The model under review builds one solid part; all positions refer to its coordinate system, in mm. Coordinates: 2 decimals unless noted, no trailing zeros. Order: outer loops, then holes, each group sorted by start corner. A loop starts at its lowest first (then second) coordinate and runs counter-clockwise, first axis right, second up. Notation, with made-up numbers: M -14.75,40 L 12.25,40 A20 ccw 12.25,51 Z; hole C 20.5,52.25 d2. An arc over 180 degrees is marked long. One line per item, written item: value.
```python
from build123d import *

# Parameters (mm, degrees)
SKETCH1_R           = 117.5
SKETCH1_R_2         = 10.25
SKETCH1_R_3         = 12.5
SKETCH1_R_4         = 1.75
BOSS_EXTRUDE1_DEPTH = 1.5


with BuildPart() as part:
    # Sketch1 → Boss-Extrude1 (new, symmetric)
    with BuildSketch(Plane(origin=(0, 0, 0), x_dir=(1, 0, 0), z_dir=(0, 1, 0))):
        with Locations(Location((0, 0, 0), (0, 0, 270))):
            Circle(SKETCH1_R)
        with Locations(Location((0, 0, 0), (0, 0, 270))):
            Circle(SKETCH1_R_2, mode=Mode.SUBTRACT)
        with Locations(Location((0, 70, 0), (0, 0, 270))):
            Circle(SKETCH1_R_3, mode=Mode.SUBTRACT)
        with Locations(Location((70, 0, 0), (0, 0, 270))):
            Circle(SKETCH1_R_3, mode=Mode.SUBTRACT)
        with Locations(Location((0, -70, 0), (0, 0, 270))):
            Circle(SKETCH1_R_3, mode=Mode.SUBTRACT)
        with Locations(Location((-70, 0, 0), (0, 0, 270))):
            Circle(SKETCH1_R_3, mode=Mode.SUBTRACT)
        with Locations(Location((0, 110, 0), (0, 0, 270))):
            Circle(SKETCH1_R_4, mode=Mode.SUBTRACT)
        with Locations(Location((77.781745931, 77.781745931, 0), (0, 0, 270))):
            Circle(SKETCH1_R_4, mode=Mode.SUBTRACT)
        with Locations(Location((110, 0, 0), (0, 0, 270))):
            Circle(SKETCH1_R_4, mode=Mode.SUBTRACT)
        with Locations(Location((77.781745931, -77.781745931, 0), (0, 0, 270))):
            Circle(SKETCH1_R_4, mode=Mode.SUBTRACT)
        with Locations(Location((0, -110, 0), (0, 0, 270))):
            Circle(SKETCH1_R_4, mode=Mode.SUBTRACT)
        with Locations(Location((-77.781745931, -77.781745931, 0), (0, 0, 270))):
            Circle(SKETCH1_R_4, mode=Mode.SUBTRACT)
        with Locations(Location((-110, 0, 0), (0, 0, 270))):
            Circle(SKETCH1_R_4, mode=Mode.SUBTRACT)
        with Locations(Location((-77.781745931, 77.781745931, 0), (0, 0, 270))):
            Circle(SKETCH1_R_4, mode=Mode.SUBTRACT)
        with Locations(Location((0, 37.5, 0), (0, 0, 270))):
            Circle(SKETCH1_R_4, mode=Mode.SUBTRACT)
        with Locations(Location((26.516504294, 26.516504294, 0), (0, 0, 270))):
            Circle(SKETCH1_R_4, mode=Mode.SUBTRACT)
        with Locations(Location((37.5, 0, 0), (0, 0, 270))):
            Circle(SKETCH1_R_4, mode=Mode.SUBTRACT)
        with Locations(Location((26.516504294, -26.516504294, 0), (0, 0, 270))):
            Circle(SKETCH1_R_4, mode=Mode.SUBTRACT)
        with Locations(Location((0, -37.5, 0), (0, 0, 270))):
            Circle(SKETCH1_R_4, mode=Mode.SUBTRACT)
        with Locations(Location((-26.516504294, -26.516504294, 0), (0, 0, 270))):
            Circle(SKETCH1_R_4, mode=Mode.SUBTRACT)
        with Locations(Location((-37.5, 0, 0), (0, 0, 270))):
            Circle(SKETCH1_R_4, mode=Mode.SUBTRACT)
        with Locations(Location((-26.516504294, 26.516504294, 0), (0, 0, 270))):
            Circle(SKETCH1_R_4, mode=Mode.SUBTRACT)
    extrude(amount=BOSS_EXTRUDE1_DEPTH, both=True)


solid = part.part
```
(1) Insertion check: pin 1 Ø5 at (x, z) = (81, -3) entering from -Y. The pin has a flat end and moves straight along its axis. Give the tip position at first contact, or say it passes through.
Geometry results:
pin 1: stops at y = -1.5
(2) We need section B-B, the plane z = -64.5. State the section outline as (x, y) points.
Geometry results:
outline: M -98.21,-1.5 L -11.22,-1.5 L -11.22,1.5 L -98.21,1.5 Z; M 11.22,-1.5 L 98.21,-1.5 L 98.21,1.5 L 11.22,1.5 Z
(3) For L1, parallel to X at y = 0.3, z = 7.5; L2, parallel to Z at x = 5, y = 0.15; L3, parallel to Z at x = 2, y = -0.5, list the stretches that pass through material, from the lowest coordinate up.
Geometry results:
L1: x = -117.26 to -80, -60 to -6.99, 6.99 to 60, 80 to 117.26
L2: z = -117.39 to -81.46, -58.54 to -8.95, 8.95 to 58.54, 81.46 to 117.39
L3: z = -117.48 to -82.34, -57.66 to -10.05, 10.05 to 57.66, 82.34 to 117.48
(4) We need section A-A, the plane x = 62.5. State the section outline as (y, z) points.
Geometry results:
outline: M -1.5,-99.5 L 1.5,-99.5 L 1.5,-10 L -1.5,-10 Z; M -1.5,10 L 1.5,10 L 1.5,99.5 L -1.5,99.5 Z
(5) Mouldability with a two-part tool opening along Z and no side actions: class faces 1 (the flat face through (-24, 1.5, -2)), 2 (the cylindrical face through (0.55, -0.021, -82.488)), 3 (the cylindrical face through (116.5, 0, -15.3)) as +Z half, -Z half, draft (parallel to the pull), parting line (faces both ways), or undercut.
Geometry results:
face 1: draft
face 2: undercut
face 3: parting line
(6) We need section C-C, the plane y = -0.95. Count the separate pieces of the cut face and the enclosed holes in it, plus the area to 3 significant figures.
Geometry results:
separate pieces: 1
enclosed holes: 21
area: 40,900 mm2
(7) We need section D-D, the plane x = -22. State the section outline as (y, z) points.
Geometry results:
outline: M -1.5,-115.42 L 1.5,-115.42 L 1.5,115.42 L -1.5,115.42 Z
